from build123d import *

# Parameters (mm, degrees)
SKETCH1_W           = 101.6
SKETCH1_H           = 63.5
BOSS_EXTRUDE1_DEPTH = 3.175
SKETCH2_R           = 3.175
CUT_EXTRUDE1_DEPTH  = 3.175
SKETCH3_R           = 2.199978507
CUT_EXTRUDE2_DEPTH  = 3.175


with BuildPart() as part:
    # Sketch1 → Boss-Extrude1 (new body)
    with BuildSketch(Plane.XY):
        with Locations((-35.329090909, 0.577272727)):
            Rectangle(SKETCH1_W, SKETCH1_H)
    extrude(amount=BOSS_EXTRUDE1_DEPTH)

    # Sketch2 → Cut-Extrude1 (cut)
    with BuildSketch(Plane.XY.offset(3.175)):
        with Locations((-77.769090909, 23.967272727)):
            Circle(SKETCH2_R)
        with Locations((7.115909091, -22.812727273)):
            Circle(SKETCH2_R)
    extrude(amount=-CUT_EXTRUDE1_DEPTH, mode=Mode.SUBTRACT)

    # Sketch3 → Cut-Extrude2 (cut)
    with BuildSketch(Plane.XY.offset(3.175)):
        with Locations((-60.499797011, 0.581401186)):
            Circle(SKETCH3_R)
    extrude(amount=-CUT_EXTRUDE2_DEPTH, mode=Mode.SUBTRACT)


solid = part.part
Geometry: final body of the model. Coordinates: model frame, mm. Coordinates: 2 decimals unless noted, no trailing zeros. Loops run counter-clockwise (first coordinate to the right, second up) from the corner with the lowest first, then second, coordinate; pieces in that order, holes last. Notation, with made-up numbers: M -23,58.5 L -12,58.5 A22 cw -12,83.5 Z; hole C 3.5,75.5 d8. An arc over 180 degrees is marked long. One line per item, written item: value. Start each with the question number.
1) Material intervals for L1, parallel to Y at x = 7.5, z = 0.25; L2, parallel to X at y = 24, z = 0.4; L3, parallel to X at y = -0.5, z = 0.9, sorted ascending. Write a range as from..to.
2) Cut plane A-A (y = -25). Return loops of the section in (x, z) (1 decimal), then the cut area to 3 significant figures.
3) Cut plane B-B (y = 25.5). Return loops of the section in (x, z) (3 decimals), then the cut area to 3 significant figures.
4) Draft query along X for faces 1 (the flat face through (-86.129, 0, 2)), 2 (the flat face through (-36, 1, 0)), 3 (the cylindrical face through (-62.698, 0.678, 1.61)), 4 (the flat face through (15.471, 0, 2)). Return one class per face: released by +X, released by -X, zero draft, split by the parting line, or undercut.
Evaluation:
1. L1: -31.17..-25.96, -19.66..32.33
1. L2: -86.13..-80.94, -74.59..15.47
1. L3: -86.13..-62.42, -58.58..15.47
2. outline: M -86.1,0 L 4.8,0 L 4.8,3.2 L -86.1,3.2 Z; M 9.4,0 L 15.5,0 L 15.5,3.2 L 9.4,3.2 Z
2. area: 308 mm^2
3. outline: M -86.129,0 L -80.55,0 L -80.55,3.175 L -86.129,3.175 Z; M -74.989,0 L 15.471,0 L 15.471,3.175 L -74.989,3.175 Z
3. area: 305 mm^2
4. face 1: released by -X
4. face 2: zero draft
4. face 3: undercut
4. face 4: released by +X
